Verification items for this drawing (mm, ordinates from the low corner). A direction names the side the tool comes from. Give positions to 0.01 mm unless a question says otherwise; leave off trailing zeros. Order: outer loops, then holes, each group sorted by start corner. A loop starts at its lowest first (then second) coordinate and runs counter-clockwise, first axis right, second up. Notation, with made-up numbers: (84.5, 69) -> (141.5, 69) arc R14 cw to (141.5, 74) -> close; hole circle Ø5 at (-8.5, -19.5). An arc over 180 degrees is marked (long way). One line per question, with ' | ' between items.
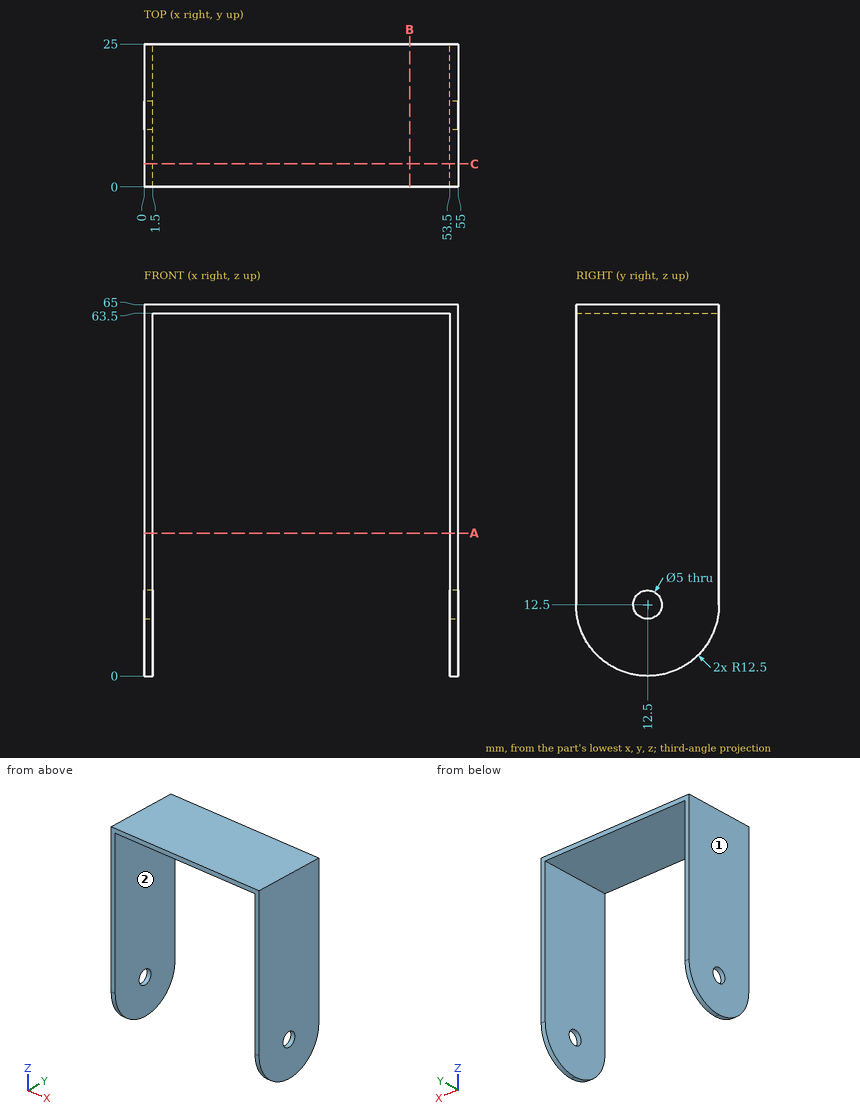
Q1. Depth check by flat-ended pin: pin 1 Ø3 at (y, z) = (12.5, 12.5) entering from +X; pin 2 Ø1 at (x, y) = (38.5, 15) entering from -Z. Enter the tip coordinate at first touch or a pass-through.
Result sheet:
pin 1: passes through | pin 2: stops at z = 63.5
Q2. Section check A-A (z = 25). Enter the section's corners in (x, y).
Result sheet:
outline: (0, 0) -> (1.5, 0) -> (1.5, 25) -> (0, 25) -> close; (53.5, 0) -> (55, 0) -> (55, 25) -> (53.5, 25) -> close
Q3. Thickness scan on line 1 (X direction, y = 7, z = 13); line 2 (Y direction, x = 0.9, z = 12.5); line 3 (Z direction, x = 36, y = 14). Record the ranges inside material, lowest first.
Result sheet:
line 1: x = 0 to 1.5, 53.5 to 55 | line 2: y = 0 to 10, 15 to 25 | line 3: z = 63.5 to 65
Q4. Access from +Z, -Z, +X, -X, +Y, -Y to the whole of each face (thin tool, end or side, straight path). Record for the marked faces 1 and 2.
Result sheet:
face 1: +Z, -Z, -X, +Y, -Y | face 2: -Z, +Y, -Y
Q5. Section check C-C (y = 4). Enter the section's corners in (x, z) (3 decimals).
Result sheet:
outline: (0, 3.335) -> (1.5, 3.335) -> (1.5, 63.5) -> (53.5, 63.5) -> (53.5, 3.335) -> (55, 3.335) -> (55, 65) -> (0, 65) -> close
Q6. Section check B-B (x = 46.5). Enter the section's corners in (y, z), and give its area (3 significant figures).
Result sheet:
outline: (0, 63.5) -> (25, 63.5) -> (25, 65) -> (0, 65) -> close | area: 37.5 mm2
